For this review, take the finished solid that the model builds, in its own axes (mm). A direction names the side the tool comes from. Round coordinates to 2 decimals unless told otherwise and drop trailing zeros. Write each loop counter-clockwise with the first axis right and the second up, starting at its lowest first coordinate (ties: lowest second). Pieces come first, ordered by that corner, then holes. Notation, with made-up numbers: (-7, -3.5) -> (38, -3.5) arc R10 ccw to (38, 11.5) -> close; hole circle Ø4 at (-19.75, 85.25). An arc over 180 degrees is marked (long way). Write each question's results on one line, items separated by ' | '. Start each with the question number.
Item 1: Add section C-C (y = 10). State the section outline as (x, z) points, plus the area to 3 significant figures.
Item 2: Clearance check with flat-ended pins moving along their axes: pin 1 (3 mm diameter, centred on x = -9.5, z = 1, fed in from -Y); pin 2 (2 mm diameter, centred on x = -25.5, z = 2, fed in from +Y); pin 3 (3 mm diameter, centred on y = -10.5, z = 1, fed in from +X). State where each tip first meets the part, or that it passes through.
Item 3: Tool access review of faces 1 (the flat face through (-15, 0, 5)), 2 (the cylindrical face through (1.02, -17.35, 2.46)), 3 (the flat face through (-0.05, 0, 2)): name each direction out of +Z, -Z, +X, -X, +Y, -Y from which nothing blocks a thin tool from reaching the whole face with its end or side.
Item 4: The part is to be moulded in two halves that separate along X. For faces 4 (the flat face through (0, -23.25, 2)), 5 (the cylindrical face through (0.98, 17.35, 2.46)), 6 (the flat face through (-34.5, 0, 2)), say which applies: +X half, -X half, draft (parallel to the pull), parting line (faces both ways), or undercut.
Item 5: To check wall thickness, follow line 1 along X through (y, z) = (5, 0.8); line 2 along Y through (x, z) = (-27, 0.5); line 3 along Y through (x, z) = (-28.5, 1.3). State the ranges of each line that lie inside material, in increasing order.
Item 6: Add section A-A (x = 1). State the section outline as (y, z) points, plus the area to 3 significant figures.
Item 7: Add section B-B (z = 1.1). State the section outline as (x, y) points.
Item 8: Add section D-D (x = -11.5). State the section outline as (y, z) points.
Autodesk Inventor part; units mm, degrees
ref_plane "YZ Plane" through (0, 0, 0) normal (1, 0, 0) x (0, 1, 0)
ref_plane "XZ Plane" through (0, 0, 0) normal (0, 1, 0) x (-1, 0, 0)
ref_plane "XY Plane" through (0, 0, 0) normal (0, 0, 1) x (1, 0, 0)
sketch "スケッチ1" plane through (0, 0, 0) normal (0, 0, 1) x (1, 0, 0)
  line L0 (0, 16.25) -> (28.4656, 16.25) construction
  line L1 (28.4656, 16.25) -> (28.4656, -16.25) construction
  line L2 (28.4656, -16.25) -> (0, -16.25) construction
  line L3 (0, -16.25) -> (0, 16.25) construction
  line L4 (5, 23.25) -> (-5.1583, 23.25)
  line L5 (-5.1583, 23.25) -> (-34.5, 15.3879)
  line L6 (-34.5, 15.3879) -> (-34.5, -15.3879)
  line L7 (-34.5, -15.3879) -> (-5.1583, -23.25)
  line L8 (-5.1583, -23.25) -> (5, -23.25)
  line L9 (5, -23.25) -> (5, -16.3)
  line L10 (5, -16.3) -> (2.05, -16.3)
  arc A0 (-0.05, -16.3) -> (2.05, -16.3) centre (1, -16.3) ccw
  line L11 (-0.05, -16.3) -> (-0.05, 16.3)
  arc A1 (2.05, 16.3) -> (-0.05, 16.3) centre (1, 16.3) ccw
  line L12 (28.4656, 0) -> (0, 0) construction
  line L13 (2.05, 16.3) -> (5, 16.3)
  line L14 (5, 16.3) -> (5, 23.25)
  line L15 (28.5156, 16.3) -> (-0.05, 16.3) construction
  line L16 (-0.05, 16.3) -> (-0.05, -16.3) construction
  line L17 (-0.05, -16.3) -> (28.5156, -16.3) construction
  line L18 (28.5156, -16.3) -> (28.5156, 16.3) construction
  circle A2 centre (-4.5, 18.25) radius 1.2
  circle A3 centre (-4.5, -18.25) radius 1.2
  line L19 (0, 0) -> (28.4656, 0) construction
  line L20 (2.5, 16.25) -> (2.5, -16.25) construction
  circle A4 centre (-4.5, 18.25) radius 5 construction
  line L21 (-6.0877, 15.5) -> (-7.6754, 18.25)
  line L22 (-7.6754, 18.25) -> (-6.0877, 21)
  line L23 (-6.0877, 21) -> (-2.9123, 21)
  line L24 (-2.9123, 21) -> (-1.3246, 18.25)
  line L25 (-1.3246, 18.25) -> (-2.9123, 15.5)
  line L26 (-2.9123, 15.5) -> (-6.0877, 15.5)
  point P0 (-34.5, 0)
  point P1 (-0.05, 0)
  dimension "d98" = 32.5
  dimension "d100" = 0.05
  dimension "d101" = 1.05
  dimension "d102" = 5
  dimension "d104" = 2.4
  dimension "d106" = 2.5
  dimension "d107" = 7
  dimension "d108" = 18.25
  dimension "d109" = 5
  dimension "d110" = 30
  dimension "d111" = 165
  dimension "d130" = 5.5
extrude "押し出し1" add sketch "スケッチ1" along normal blind 5 contours L14 L13 A1 L11 A0 L10 L9 L8 L7 L6 L5 L4 | L21 L22 L23 L24 L25 L26
sketch "スケッチ8" plane through (0, 0, 0) normal (0, 0, -1) x (-1, 0, 0)
  circle A0 centre (4.5, 18.25) radius 1.2
  circle A1 centre (4.5, 18.25) radius 1.2
  circle A2 centre (4.5, -18.25) radius 1.2
  circle A3 centre (4.5, -18.25) radius 1.2
  point P0 (0, 0)
extrude "押し出し6" add sketch "スケッチ8" against normal up to surface (5 mm away)
properties part number "胴体_サブフレーム_1_7" material "アセタール樹脂、黒"
Responses:
1) outline: (-34.5, 0) -> (-0.05, 0) -> (-0.05, 5) -> (-34.5, 5) -> close | area: 172 mm^2
2) pin 1: stops at y = -22.49 | pin 2: stops at y = 18.07 | pin 3: stops at x = -0.05
3) face 1: +Z, +X, -X, +Y, -Y | face 2: +Z, -Z | face 3: +Z, -Z, +X
4) face 4: draft | face 5: undercut | face 6: -X half
5) line 1: x = -34.5 to -0.05 | line 2: y = -17.4 to 17.4 | line 3: y = -17 to 17
6) outline: (-23.25, 0) -> (-17.35, 0) -> (-17.35, 5) -> (-23.25, 5) -> close; (17.35, 0) -> (23.25, 0) -> (23.25, 5) -> (17.35, 5) -> close | area: 59.0 mm^2
7) outline: (-34.5, -15.39) -> (-5.16, -23.25) -> (5, -23.25) -> (5, -16.3) -> (2.05, -16.3) arc R1.05 cw to (-0.05, -16.3) -> (-0.05, 16.3) arc R1.05 cw to (2.05, 16.3) -> (5, 16.3) -> (5, 23.25) -> (-5.16, 23.25) -> (-34.5, 15.39) -> close
8) outline: (-21.55, 0) -> (21.55, 0) -> (21.55, 5) -> (-21.55, 5) -> close
